Here's how the part is built. I have some questions about the finished solid (model axes, mm). Face numbers are marked on the shaded views. A direction names the side the tool comes from. Give positions to 0.01 mm unless a question says otherwise; leave off trailing zeros. Write each loop counter-clockwise with the first axis right and the second up, starting at its lowest first coordinate (ties: lowest second). Pieces come first, ordered by that corner, then holes. Notation, with made-up numbers: (79.25, 56.5) -> (115.25, 56.5) arc R32 ccw to (115.25, 86.5) -> close; hole circle Ø3 at (85, 85.5). An arc over 180 degrees is marked (long way). Return JSON: item names as keys, results as strings.
from build123d import *

# Parameters (mm, degrees)
F1_DEPTH  = 28.575
F2_START  = 3.175
F2_DEPTH  = 22.225
F3_START  = 3.175
F0_W      = 38.1
F0_H      = 15.875
F3_DEPTH  = 22.225
F5_DEPTH  = 19.05
F6_R      = 6.35
F7_START  = 9.525
F0_W_2    = 6.35
F0_H_2    = 4.6355
F7_DEPTH  = 9.525
F8_R      = 2.54
F9_R      = 2.5796875
F10_DEPTH = 47.626


with BuildPart() as f1:
    # F0 (on Top) → F1 (new body)
    with BuildSketch(Plane.XY):
        with BuildLine():
            Line((0, 127), (0, 92.075))
            ThreePointArc((0, 92.075), (5.5775580758, 91.6267526155), (11.0119450237, 90.2935165876))
            Line((11.0119450237, 90.2935165876), (0, 127))
        make_face()
        with BuildLine():
            ThreePointArc((-11.0119450237, 90.2935165876), (-5.5775580758, 91.6267526155), (0, 92.075))
            Line((0, 92.075), (0, 127))
            Line((0, 127), (-11.0119450237, 90.2935165876))
        make_face()
    extrude(amount=F1_DEPTH)



with BuildPart() as f1b:
    # F0 (on Top) → F1, piece 2 (new body)
    with BuildSketch(Plane.XY):
        with BuildLine():
            Line((0, 22.225), (0, 0))
            Line((0, 0), (38.1, 0))
            Line((38.1, 0), (27.4375962607, 35.5413457977))
            ThreePointArc((27.4375962607, 35.5413457977), (15.2491536976, 25.7299596355), (0, 22.225))
        make_face()
        with BuildLine():
            Line((-38.1, 0), (0, 0))
            Line((0, 0), (0, 22.225))
            ThreePointArc((0, 22.225), (-15.2491536976, 25.7299596355), (-27.4375962607, 35.5413457977))
            Line((-27.4375962607, 35.5413457977), (-38.1, 0))
        make_face()
        with BuildLine():
            Line((-38.1, -6.35), (-38.1, 0))
            Line((-38.1, 0), (-27.4375962607, 35.5413457977))
            ThreePointArc((-27.4375962607, 35.5413457977), (-34.7126867768, 53.3048729883), (-31.5015963811, 72.2299552534))
            Line((-31.5015963811, 72.2299552534), (-50.8, 88.9))
            Line((-50.8, 88.9), (-50.8, 73.025))
            Line((-50.8, 73.025), (-50.8, 38.1))
            Line((-50.8, 38.1), (-50.8, 3.175))
            Line((-50.8, 3.175), (-50.8, -6.35))
            Line((-50.8, -6.35), (-38.1, -6.35))
        make_face()
        Polygon((-107.95, 3.175), (-50.8, 3.175), (-50.8, 38.1), (-107.95, 38.1), (-107.95, 25.273), (-107.95, 20.6375), (-107.95, 16.002), align=None)
    extrude(amount=F1_DEPTH)


with BuildPart() as f1_1:
    add(f1.part)

    add(f1b.part)  # F2 merges F1b
    # F0 (on Top) → F2 (join)
    with BuildSketch(Plane.XY.offset(F2_START)):
        with BuildLine():
            ThreePointArc((-31.5015963811, 72.2299552534), (-34.7126867768, 53.3048729883), (-27.4375962607, 35.5413457977))
            Line((-27.4375962607, 35.5413457977), (-11.0119450237, 90.2935165876))
            ThreePointArc((-11.0119450237, 90.2935165876), (-23.0959598786, 83.3479438561), (-31.5015963811, 72.2299552534))
        make_face()
        with BuildLine():
            ThreePointArc((-27.4375962607, 35.5413457977), (-15.2491536976, 25.7299596355), (0, 22.225))
            Line((0, 22.225), (0, 92.075))
            ThreePointArc((0, 92.075), (-5.5775580758, 91.6267526155), (-11.0119450237, 90.2935165876))
            Line((-11.0119450237, 90.2935165876), (-27.4375962607, 35.5413457977))
        make_face()
        with BuildLine():
            Line((0, 92.075), (0, 22.225))
            ThreePointArc((0, 22.225), (15.2491536976, 25.7299596355), (27.4375962607, 35.5413457977))
            Line((27.4375962607, 35.5413457977), (11.0119450237, 90.2935165876))
            ThreePointArc((11.0119450237, 90.2935165876), (5.5775580758, 91.6267526155), (0, 92.075))
        make_face()
        with BuildLine():
            Line((11.0119450237, 90.2935165876), (27.4375962607, 35.5413457977))
            ThreePointArc((27.4375962607, 35.5413457977), (33.0001035938, 45.71545638), (34.925, 57.15))
            ThreePointArc((34.925, 57.15), (28.3226747056, 77.5848164299), (11.0119450237, 90.2935165876))
        make_face()
    extrude(amount=F2_DEPTH)

    # F0 (on Top) → F3 (join)
    with BuildSketch(Plane.XY.offset(F3_START)):
        with Locations((-69.85, 80.9625)):
            Rectangle(F0_W, F0_H)
    extrude(amount=F3_DEPTH)

    # F4 (on face) → F5 (join, symmetric)
    with BuildSketch(Plane.XY):
        with BuildLine():
            ThreePointArc((0, 49.0477367043), (5.6126600757, 51.3725766287), (7.9375, 56.9852367043))
            ThreePointArc((7.9375, 56.9852367043), (5.6126600757, 62.59789678), (0, 64.9227367043))
            Line((0, 64.9227367043), (0, 49.0477367043))
        make_face()
        with BuildLine():
            Line((0, 49.0477367043), (0, 64.9227367043))
            ThreePointArc((0, 64.9227367043), (-7.9375, 56.9852367043), (0, 49.0477367043))
        make_face()
    extrude(amount=F5_DEPTH, both=True)

    # F6
    f6_edges = [f1_1.edges().sort_by_distance(p)[0] for p in [
        (0, 127, 14.2875),
        (38.1, 0, 14.2875),
        (-107.95, 3.175, 14.2875),
        (-107.95, 38.1, 14.2875),
    ]]
    fillet(f6_edges, radius=F6_R)

    # F0 (on Top) → F7 (join)
    with BuildSketch(Plane.XY.offset(F7_START)):
        with Locations((-111.125, 22.95525)):
            Rectangle(F0_W_2, F0_H_2)
        with Locations((-111.125, 18.31975)):
            Rectangle(F0_W_2, F0_H_2)
    extrude(amount=F7_DEPTH)

    # F8
    f8_edges = [f1_1.edges().sort_by_distance(p)[0] for p in [
        (-111.125, 25.273, 19.05),
        (-111.125, 16.002, 19.05),
        (-111.125, 16.002, 9.525),
        (-111.125, 25.273, 9.525),
    ]]
    fillet(f8_edges, radius=F8_R)

    # F9 (on face) → F10 (cut, through all)
    with BuildSketch(Plane.XY.offset(28.575)):
        with Locations((0, 104.775)):
            Circle(F9_R)
        with Locations((28.965945942, 5.3702991543)):
            Circle(F9_R)
        with Locations((-30.5421855315, 5.3702991543)):
            Circle(F9_R)
    extrude(amount=-F10_DEPTH, mode=Mode.SUBTRACT)


solid = f1_1.part
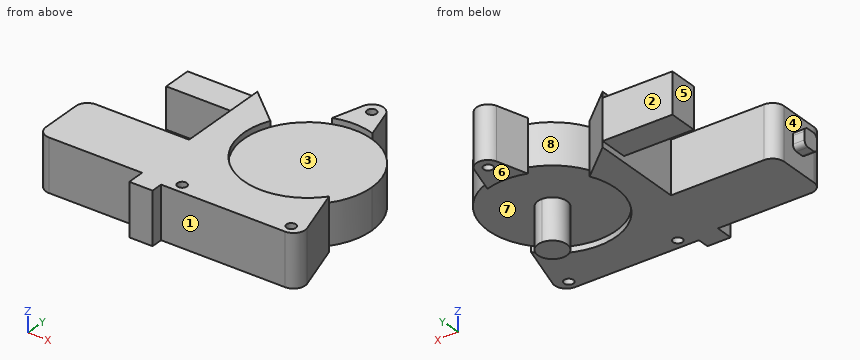
1. For pin 1 Ø1 at (x, z) = (-28.5, 8) entering from +Y; pin 2 Ø6 at (y, z) = (90.5, 2.5) entering from -X; pin 3 Ø2 at (x, y) = (-112, 20) entering from -Z (3 decimals), each with a flat end and sliding along its axis, tell me the tip position at first contact or that it passes through.
Taken from the geometry:
{"pin 1": "stops at y = 78.02", "pin 2": "stops at x = -88.9", "pin 3": "stops at z = 9.525"}
2. Suppose I cut it at A-A, the plane y = 83. List the corners of the cut face in (x, z) for me (3 decimals).
Taken from the geometry:
{"outline": "(-88.9, 3.175) -> (-50.8, 3.175) -> (-50.8, 0) -> (-43.97, 0) -> (-43.97, 28.575) -> (-50.8, 28.575) -> (-50.8, 25.4) -> (-88.9, 25.4) -> close; (-23.485, 3.175) -> (23.485, 3.175) -> (23.485, 25.4) -> (-23.485, 25.4) -> close"}
3. If I drill on line 1 (Y direction, x = 0, z = 7.5); line 2 (Z direction, x = -27, y = 74.5) (3 decimals); line 3 (X direction, y = 75.5, z = 6), over which ranges is the centre line in solid material (lowest first)? Write a range as [from, to].
Taken from the geometry:
{"line 1": "y = [0, 102.2], [107.35, 111.25]", "line 2": "z = [3.175, 25.4]", "line 3": "x = [-88.9, -35.29], [-29.72, 29.72]"}
4. Suppose I cut it at D-D, the plane z = -13. List the corners of the cut face in (x, y) for me (1 decimal).
Taken from the geometry:
{"outline": "circle Ø15.9 at (0, 57)"}
5. Which directions (+Z, -Z, +X, -X, +Y, -Y) give clear straight access to the entire face, cutting with the end or side of a thin tool? Please do the marked faces 1, 2, 3 and 4.
Taken from the geometry:
{"face 1": "+Z, -Z, +X, -Y", "face 2": "+Z, -Z, -X, +Y", "face 3": "+Z", "face 4": "-X"}
6. Suppose I cut it at B-B, the plane z = 21.5. Count the separate pieces of the cut face and the enclosed holes in it, and give its area (3 significant figures).
Taken from the geometry:
{"separate pieces": "1", "enclosed holes": "3", "area": "9,980 mm²"}
7. Suppose I cut it at C-C, the plane x = -25. List the corners of the cut face in (y, z) for me (3 decimals), and give its area (3 significant figures).
Taken from the geometry:
{"outline": "(0, 0) -> (32.762, 0) -> (32.762, 3.175) -> (81.538, 3.175) -> (81.538, 25.4) -> (32.762, 25.4) -> (32.762, 28.575) -> (0, 28.575) -> close", "area": "2,020 mm²"}
8. If we mould it in two halves opening along X, with no side actions, what happens to the marked faces 5, 6, 7 and 8? For each: released by +X, released by -X, zero draft, split by the parting line, or undercut.
Taken from the geometry:
{"face 5": "released by -X", "face 6": "zero draft", "face 7": "undercut", "face 8": "undercut"}
